```python
from build123d import *

# Parameters (mm, degrees)
SKETCH1_R           = 8
BOSS_EXTRUDE1_DEPTH = 3.175


with BuildPart() as part:
    # Sketch1 → Boss-Extrude1 (new body)
    with BuildSketch(Plane.XY):
        Polygon((45.481871178, 132.088945011), (37.212440054, 108.072773191), (40.214461532, 107.039094301), (34.01238819, 89.026965435), (31.010366712, 90.060644326), (24.80829337, 72.048515461), (27.810314847, 71.01483657), (21.608241505, 53.002707705), (18.606220027, 54.036386596), (12.404146685, 36.02425773), (15.406168162, 34.99057884), (9.20409482, 16.978449975), (6.202073342, 18.012128865), (0, 0), (9.97035014, -12.312357038), (12.437788568, -10.314264796), (24.426342017, -25.118895362), (21.95890359, -27.116987604), (41.939826006, -51.79137188), (44.407264433, -49.793279638), (56.395817883, -64.597910204), (53.928379455, -66.596002446), (55.946582764, -69.088275974), (152.4, 0), (152.4, 3.175), (133.35, 3.175), (133.35, 0), (120.65, 0), (120.65, 3.175), (95.25, 3.175), (95.25, 0), (82.55, 0), (82.55, 3.175), (57.15, 3.175), (57.15, 0), (44.45, 0), (44.45, 3.175), (44.45, 66.675), (101.6, 66.675), (101.6, 128.913945011), (82.55, 128.913945011), (82.55, 132.088945011), align=None)
        with Locations((38.1, -12.7)):
            Circle(SKETCH1_R, mode=Mode.SUBTRACT)
    extrude(amount=BOSS_EXTRUDE1_DEPTH)


solid = part.part
```
Geometry: final body of the model. Coordinates: model frame, mm. Round coordinates to 2 decimals unless told otherwise and drop trailing zeros. Order: outer loops, then holes, each group sorted by start corner. A loop starts at its lowest first (then second) coordinate and runs counter-clockwise, first axis right, second up. Notation, with made-up numbers: M -24.75,-9 L 6.25,-9 A24 cw 6.25,2 Z; hole C 61,-34.75 d6. An arc over 180 degrees is marked long. Use one line per item in the form item = value. Start each with the question number.
Q1. Cut plane A-A (x = 76.5). Return loops of the section in (y, z) (3 decimals).
Q2. Cut plane B-B (y = 82.5). Return loops of the section in (x, z) (3 decimals), and give its area (3 significant figures).
Q3. Pin query (flat end, axial travel): pin 1 Ø1 at (y, z) = (2, 1) entering from -X; pin 2 Ø1.5 at (y, z) = (81.5, 1) entering from -X; pin 3 Ø1.6 at (x, z) = (78, 1.5) entering from -Y; pin 4 Ø10 at (x, y) = (93, 86.5) entering from -Z. Return the tip coordinate at first contact, or that it passes through.
Q4. Material intervals for line 1 (Y direction, x = 59, z = 1.5) (3 decimals); line 2 (Y direction, x = 83.5, z = 0.5) (3 decimals); line 3 (Y direction, x = 116.5, z = 2.45) (3 decimals), sorted ascending. Write a range as [from, to].
Q5. Cut plane C-C (y = 111). Return loops of the section in (x, z) (3 decimals), and give its area (3 significant figures).
Q6. Mould query, pull axis Y, two halves, no side actions, for faces 1 (the face through (4.915, -6.07, 1.565)), 2 (the face through (42, 32, 3.175)), 3 (the face through (30.108, -12.348, 1.565)). Classes: +Y half, -Y half, draft (parallel to the pull), parting line (faces both ways), or undercut.
Geometry results:
q1.outline = M -54.366,0 L 3.175,0 L 3.175,3.175 L -54.366,3.175 Z; M 66.675,0 L 132.089,0 L 132.089,3.175 L 66.675,3.175 Z
q2.outline = M 28.407,0 L 101.6,0 L 101.6,3.175 L 28.407,3.175 Z
q2.area = 232 mm^2
q3.pin_1 = 0.52
q3.pin_2 = 27.8
q3.pin_3 = -53.86
q3.pin_4 = 0
q4.line_1 = [-66.901, 3.175], [66.675, 132.089]
q4.line_2 = [-49.352, 0], [66.675, 128.914]
q4.line_3 = [-25.715, 3.175]
q5.outline = M 38.22,0 L 101.6,0 L 101.6,3.175 L 38.22,3.175 Z
q5.area = 201 mm^2
q6.face_1 = -Y half
q6.face_2 = draft
q6.face_3 = undercut
